Source: three-view drawing plus pictorial views. Frame: mm from the lowest corner of the part. A direction names the side the tool comes from. Give positions to 0.01 mm unless a question says otherwise; leave off trailing zeros. Order: outer loops, then holes, each group sorted by start corner. A loop starts at its lowest first (then second) coordinate and runs counter-clockwise, first axis right, second up. Notation, with made-up numbers: (51, -1.75) -> (88, -1.75) arc R28 ccw to (88, 32.25) -> close; hole circle Ø6 at (3, -37). An arc over 180 degrees is marked (long way). Answer in a Markdown table with one row per item.
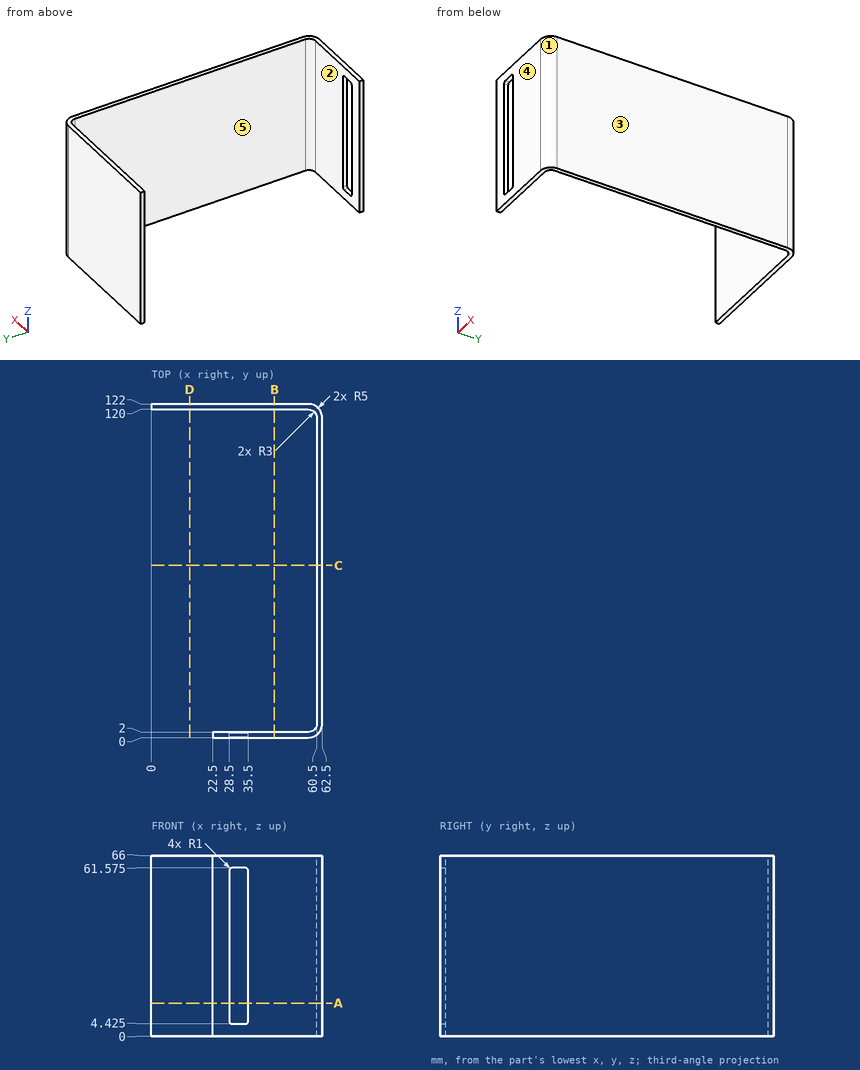
(1) Section query C-C (y = 63). Return the cut outline in (x, z).
A:
| item | result |
|---|---|
| outline | (60.5, 0) -> (62.5, 0) -> (62.5, 66) -> (60.5, 66) -> close |
(2) First-contact query: pin 1 Ø2 at (y, z) = (0.5, 37) entering from +X; pin 2 Ø10 at (x, z) = (14.5, 36) entering from -Y; pin 3 Ø2 at (y, z) = (0.5, 48.5) entering from -X. Flat tips, straight axial feed; report the tip coordinate or a pass-through.
A:
| item | result |
|---|---|
| pin 1 | stops at x = 61.07 |
| pin 2 | stops at y = 120 |
| pin 3 | stops at x = 22.5 |
(3) Ray query, probe 1 along Y at (x, z) = (24, 39.5); probe 2 along Y at (x, z) = (16, 57.5); probe 3 along X at (y, z) = (82.5, 37). Return the intervals inside material, ascending.
A:
| item | result |
|---|---|
| probe 1 | y = 0 to 2, 120 to 122 |
| probe 2 | y = 120 to 122 |
| probe 3 | x = 60.5 to 62.5 |
(4) Pull-direction query (Y, two-part tool) for the marked faces 1, 2 and 3; classes: +Y half, -Y half, draft (parallel to the pull), parting line (faces both ways), or undercut.
A:
| item | result |
|---|---|
| face 1 | -Y half |
| face 2 | undercut |
| face 3 | draft |
(5) Section query B-B (x = 45). Return the cut outline in (y, z).
A:
| item | result |
|---|---|
| outline | (0, 0) -> (2, 0) -> (2, 66) -> (0, 66) -> close; (120, 0) -> (122, 0) -> (122, 66) -> (120, 66) -> close |
(6) Section query D-D (x = 14). Return the cut outline in (y, z).
A:
| item | result |
|---|---|
| outline | (120, 0) -> (122, 0) -> (122, 66) -> (120, 66) -> close |
(7) Access query for the marked faces 4 and 5. Directions: +Z, -Z, +X, -X, +Y, -Y. A direction counts if a zero-diameter tool reaches every point of the face in a straight line with its end or side. Return the directions, or none.
A:
| item | result |
|---|---|
| face 4 | +Z, -Z, +X, -X, -Y |
| face 5 | +Z, -Z, -X |
(8) Section query A-A (z = 12). Return the cut outline in (x, y).
A:
| item | result |
|---|---|
| outline | (0, 120) -> (57.5, 120) arc R3 cw to (60.5, 117) -> (60.5, 5) arc R3 cw to (57.5, 2) -> (35.5, 2) -> (35.5, 0) -> (57.5, 0) arc R5 ccw to (62.5, 5) -> (62.5, 117) arc R5 ccw to (57.5, 122) -> (0, 122) -> close; (22.5, 0) -> (28.5, 0) -> (28.5, 2) -> (22.5, 2) -> close |
